The listing builds one solid part. Answer for the finished solid, in the listing's coordinates (mm). A direction names the side the tool comes from. Coordinates: 2 decimals unless noted, no trailing zeros. Write item = value, one per line.
from build123d import *

# Parameters (mm, degrees)
SKETCH_1_W          = 60
SKETCH_1_H          = 45.5
EXTRUDE_1_DEPTH     = 2
SKETCH_2_W          = 7
SKETCH_2_H          = 2
SKETCH_2_W_2        = 2
SKETCH_2_H_2        = 7
CUT_EXTRUDE_1_DEPTH = 76.327617777
SKETCH_4_R          = 0.5
CUT_EXTRUDE_2_DEPTH = 76.327617777
SKETCH_5_W          = 20.5
SKETCH_5_H          = 8
CUT_EXTRUDE_3_DEPTH = 76.327617777
SKETCH_6_W          = 6.5
SKETCH_6_H          = 5
EXTRUDE_2_DEPTH     = 2
SKETCH_7_R          = 0.5
CUT_EXTRUDE_4_DEPTH = 76.327617777
SKETCH_8_W          = 19.5
SKETCH_8_H          = 2.5
CUT_EXTRUDE_5_DEPTH = 76.327617777
FILLET_1_R          = 1
SKETCH_9_R          = 0.5
CUT_EXTRUDE_6_DEPTH = 2
SKETCH_10_R         = 1.5
CUT_EXTRUDE_7_DEPTH = 76.327617777


with BuildPart() as part:
    # 草图1 → 凸台-拉伸1 (new body)
    with BuildSketch(Plane.XY):
        with Locations((30, 22.75)):
            Rectangle(SKETCH_1_W, SKETCH_1_H)
    extrude(amount=EXTRUDE_1_DEPTH)

    # 草图2 → 切除-拉伸1 (cut, through all)
    with BuildSketch(Plane.XY.offset(2)):
        with Locations((9.5, 44.5)):
            Rectangle(SKETCH_2_W, SKETCH_2_H)
        with Locations((43.75, 44.5)):
            Rectangle(SKETCH_2_W, SKETCH_2_H)
        with Locations((15.5, 1)):
            Rectangle(SKETCH_2_W, SKETCH_2_H)
        with Locations((37.5, 1)):
            Rectangle(SKETCH_2_W, SKETCH_2_H)
        with Locations((1, 32)):
            Rectangle(SKETCH_2_W_2, SKETCH_2_H_2)
        with Locations((1, 13.5)):
            Rectangle(SKETCH_2_W_2, SKETCH_2_H_2)
        with Locations((59, 32)):
            Rectangle(SKETCH_2_W_2, SKETCH_2_H_2)
        with Locations((59, 13.5)):
            Rectangle(SKETCH_2_W_2, SKETCH_2_H_2)
    extrude(amount=-CUT_EXTRUDE_1_DEPTH, mode=Mode.SUBTRACT)

    # 草图4 → 切除-拉伸2 (cut, through all)
    with BuildSketch(Plane.XY.offset(2)):
        with Locations((6, 43.5)):
            Circle(SKETCH_4_R)
    cut_extrude_2 = extrude(amount=-CUT_EXTRUDE_2_DEPTH, mode=Mode.SUBTRACT)

    # 草图5 → 切除-拉伸3 (cut, through all)
    with BuildSketch(Plane.XY.offset(2)):
        with Locations((25.75, 25.5)):
            Rectangle(SKETCH_5_W, SKETCH_5_H)
    extrude(amount=-CUT_EXTRUDE_3_DEPTH, mode=Mode.SUBTRACT)

    # 草图6 → 凸台-拉伸2 (add)
    with BuildSketch(Plane.XY.offset(2)):
        with Locations((18.75, 24)):
            Rectangle(SKETCH_6_W, SKETCH_6_H)
        with Locations((32.75, 24)):
            Rectangle(SKETCH_6_W, SKETCH_6_H)
    extrude(amount=-EXTRUDE_2_DEPTH)

    # 草图7 → 切除-拉伸4 (cut, through all)
    with BuildSketch(Plane.XY.offset(2)):
        with Locations((15.5, 29.5)):
            Circle(SKETCH_7_R)
        with Locations((15.5, 26.5)):
            Circle(SKETCH_7_R)
        with Locations((36, 29.5)):
            Circle(SKETCH_7_R)
        with Locations((36, 26.5)):
            Circle(SKETCH_7_R)
    extrude(amount=-CUT_EXTRUDE_4_DEPTH, mode=Mode.SUBTRACT)

    # 草图8 → 切除-拉伸5 (cut, through all)
    with BuildSketch(Plane.XY.offset(2)):
        with Locations((25.75, 21.25)):
            Rectangle(SKETCH_8_W, SKETCH_8_H)
    extrude(amount=-CUT_EXTRUDE_5_DEPTH, mode=Mode.SUBTRACT)

    # 圆角1
    fillet_1_edges = [part.edges().sort_by_distance(p)[0] for p in [
        (22, 26.5, 1),
        (29.5, 26.5, 1),
        (29.5, 22.5, 1),
        (22, 22.5, 1),
    ]]
    fillet(fillet_1_edges, radius=FILLET_1_R)

    # 草图阵列1: 切除-拉伸2 at 15 more places
    with Locations((7, 0, 0), (34.25, 0, 0), (41.25, 0, 0), (6, -41.5, 0), (13, -41.5, 0), (28, -41.5, 0), (35, -41.5, 0), (-4, -8, 0), (-4, -15, 0), (-4, -26.5, 0), (-4, -33.5, 0), (52, -8, 0), (52, -15, 0), (52, -26.5, 0), (52, -33.5, 0)):
        add(cut_extrude_2, mode=Mode.SUBTRACT)

    # 草图9 → 切除-拉伸6 (cut)
    with BuildSketch(Plane.XY.offset(2)):
        with Locations((16, 20)):
            Circle(SKETCH_9_R)
        with Locations((16, 22.5)):
            Circle(SKETCH_9_R)
        with Locations((35.5, 20)):
            Circle(SKETCH_9_R)
        with Locations((35.5, 22.5)):
            Circle(SKETCH_9_R)
    extrude(amount=-CUT_EXTRUDE_6_DEPTH, mode=Mode.SUBTRACT)

    # 草图10 → 切除-拉伸7 (cut, through all)
    with BuildSketch(Plane.XY.offset(2)):
        with Locations((20.5, 20)):
            Circle(SKETCH_10_R)
    extrude(amount=-CUT_EXTRUDE_7_DEPTH, mode=Mode.SUBTRACT)


solid = part.part
Q1. A tool of negligible diameter and unlimited length cuts with its end or side. For faces 1 (the face through (59, 10, 1)), 2 (the face through (37, 2, 1)), 3 (the face through (36, 28, 1)), from which of +Z, -Z, +X, -X, +Y, -Y can it reach the whole face along a straight path? Write none if from no direction.
The answers:
face_1 = +Z, -Z, +X
face_2 = +Z, -Z, -Y
face_3 = +Z, -Z
Q2. Find the intervals of material crossed by line 1 along Y through (x, z) = (23, 1.55); line 2 along X through (y, z) = (25.5, 1.45); line 3 along X through (y, z) = (12.5, 1.6), in increasing order.
The answers:
line_1 = 0 to 20, 29.5 to 45.5
line_2 = 0 to 22, 29.5 to 60
line_3 = 2 to 58
Q3. This flat-tipped pin is pushed along its axis until it touches: pin 1 Ø0.6 at (x, z) = (36, 1) entering from -Y. Where does it stop, or does it pass through?
The answers:
pin_1 = 2
Q4. The mould has two halves that part along X. Classify faces 4 (the face through (0, 5, 1)), 5 (the face through (47.25, 45, 1)), 6 (the face through (34, 1, 1)), 7 (the face through (59, 35.5, 1)): released by +X, released by -X, zero draft, split by the parting line, or undercut.
The answers:
face_4 = released by -X
face_5 = undercut
face_6 = undercut
face_7 = zero draft
